Can you work these out from the model? Positions are in its coordinate system, mm. A direction names the side the tool comes from. Coordinates: 2 decimals unless noted, no trailing zeros. Loops run counter-clockwise (first coordinate to the right, second up) from the corner with the lowest first, then second, coordinate; pieces in that order, holes last.
Autodesk Fusion 360 part; units mm, degrees
sketch "草图1" plane through (0, 0, 0) normal (0, 1, 0) x (1, 0, 0)
  line L0 (-100, 0) -> (100, 0) construction
  line L1 (-50, 0) -> (-50, -14)
  line L2 (-50, -14) -> (-26.533, -14)
  arc A0 (-26.533, -14) -> (26.533, -14) centre (0, 0) ccw
  line L3 (26.533, -14) -> (50, -14)
  line L4 (50, -14) -> (50, 0)
  line L5 (18, 0) -> (50, 0)
  line L6 (-50, 0) -> (-18, 0)
  line L7 (0, -85) -> (0, 30) construction
  arc A1 (-18, 0) -> (18, 0) centre (0, 0) ccw
  circle A2 centre (0, -60) radius 16
  circle A3 centre (0, -60) radius 9
  line L8 (-26.533, -14) -> (-15.6243, -63.4469)
  line L9 (26.533, -14) -> (15.6243, -63.4469)
  line L10 (-21.2383, -38) -> (21.2383, -38)
  dimension "d1" = 14
  dimension "d2" = 14
  dimension "d3" = 100
  dimension "d5" = 30
  dimension "d6" = 18
  dimension "d7" = 32
  dimension "d8" = 18
  dimension "d9" = 60
  dimension "d10" = 38
extrude "拉伸1" add sketch "草图1" against normal blind 50 contours L1 L2 A0 L3 L4 L5 L6 A1 makes body 1
extrude "拉伸2" add sketch "草图1" against normal blind 45 contours A0 L8 L9 L10 bodies 1
extrude "拉伸3" add sketch "草图1" against normal blind 15 contours A2 L8 L9 L10 bodies 1
extrude "拉伸4" add sketch "草图1" against normal blind 17 contours A2 bodies 1
sketch "草图2" plane through (0, 0, 0) normal (1, 0, 0) x (0, 1, 0)
  line L0 (-15, 63.4469) -> (-15, 41)
  line L1 (-18, 38) -> (-45, 38)
  arc A0 (-18, 38) -> (-15, 41) centre (-18, 41) ccw
  line L2 (-15, 63.4469) -> (-15, 38)
  line L3 (-15, 38) -> (-45, 38)
  point P0 (-15, 63.4469)
  point P1 (-45, 38)
  point P2 (-15, 38)
  dimension "d19" = 3
extrude "拉伸5" add sketch "草图2" along normal mid plane 54 separate body makes body 2
extrude "拉伸6" cut sketch "草图1" against normal blind 75 contours A2 L8 L9 L10 keep common part bodies 2
combine "合并1" operation add target body 1 tool bodies 2
sketch "草图3" plane through (0, 0, 0) normal (0, 0, 1) x (1, 0, 0)
  line L0 (-50, -17) -> (-50, -33)
  line L1 (-50, -33) -> (-36, -33)
  arc A0 (-36, -33) -> (-36, -17) centre (-36, -25) ccw
  line L2 (-36, -17) -> (-50, -17)
  line L3 (0, 15) -> (0, -36) construction
  line L4 (36, -17) -> (50, -17)
  line L5 (50, -17) -> (50, -33)
  line L6 (50, -33) -> (36, -33)
  arc A1 (36, -17) -> (36, -33) centre (36, -25) ccw
  dimension "d24" = 50
  dimension "d25" = 36
  dimension "d26" = 16
  dimension "d27" = 25
extrude "拉伸7" cut sketch "草图3" along normal blind 14 bodies 1
sketch "草图4" plane through (0, 0, 38) normal (0, 0, 1) x (-1, 0, 0)
  line L0 (-21.2383, 18) -> (21.2383, 18)
  line L1 (21.2383, 18) -> (21.2383, 45)
  line L2 (21.2383, 45) -> (-21.2383, 45)
  line L3 (-21.2383, 45) -> (-21.2383, 18)
  circle A0 centre (0, 30) radius 5
  line L4 (0, 45) -> (0, 18) construction
  dimension "d30" = 15
  dimension "d31" = 10
extrude "拉伸8" cut sketch "草图4" against normal blind 57 contours A0 bodies 1
equation "d10 = 60 mm - 22 mm"
(1) I want a section at A-A on x = -40. Write out the boundary of the cut face in (y, z).
Check values:
outline: (-50, 0) - (-33, 0) - (-33, 14) - (-50, 14) - close; (-17, 0) - (0, 0) - (0, 14) - (-17, 14) - close
(2) I want a section at C-C on z = 60. Write out the boundary of the cut face in (x, y), then the cut area to 3 significant figures.
Check values:
outline: (-16.38, -15) - (-16, -15) - (-16, -17) - (-9, -17) - (-9, 0) - (-16.38, 0) - close; (9, -17) - (16, -17) - (16, -15) - (16.38, -15) - (16.38, 0) - (9, 0) - close
area: 250 mm2
(3) I want a section at D-D on y = -30. Write out the boundary of the cut face in (x, z) (3 decimals).
Check values:
outline: (-29.755, 0) - (-18, 0) arc R18 cw to (-5, 17.292) - (-5, 38) - (-21.238, 38) - (-26.533, 14) - (-29.755, 14) - close; (5, 17.292) arc R18 cw to (18, 0) - (29.755, 0) - (29.755, 14) - (26.533, 14) - (21.238, 38) - (5, 38) - close
(4) I'm going to push flat-ended pins straight in: pin 1 (23.5 mm diameter, centred on x = 0, z = 60, fed in from -Y); pin 2 (7 mm diameter, centred on x = 37, y = -18, fed in from +Z); pin 3 (2 mm diameter, centred on y = -15.5, z = 65, fed in from -X); pin 4 (1 mm diameter, centred on x = 16, z = 66, fed in from +Y). Where does each tip first touch, or does it pass through?
Check values:
pin 1: stops at y = -17
pin 2: stops at z = 14
pin 3: stops at x = -15.49
pin 4: passes through
(5) Which directions (+Z, -Z, +X, -X, +Y, -Y) give clear straight access to the entire face, cutting with the end or side of a thin tool? Please do faces 1 (the flat face through (30, -19, 14)), 2 (the flat face through (-38, -14, 14)), 3 (the cylindrical face through (-3.47, -8.38, 75.62)), 4 (the flat face through (-5, -31.3, 38)).
Check values:
face 1: +Z, +X, +Y, -Y
face 2: +Z, -X, +Y, -Y
face 3: -Y
face 4: +Z, +X, -X, -Y
(6) I want a section at B-B on x = 0. Write out the boundary of the cut face in (y, z).
Check values:
outline: (-50, 18) - (-35, 18) - (-35, 38) - (-45, 38) - (-45, 30) - (-50, 30) - close; (-25, 18) - (0, 18) - (0, 51) - (-17, 51) - (-17, 44) - (-15, 44) - (-15, 41) arc R3 cw to (-18, 38) - (-25, 38) - close; (-17, 69) - (0, 69) - (0, 76) - (-17, 76) - close
(7) If we mould it in two halves opening along Y, with no side actions, what happens to faces 5 (the cylindrical face through (28, -25, 7)), 6 (the flat face through (0, -45, 31)), 7 (the flat face through (50, -8, 7))? For each: released by +Y, released by -Y, zero draft, split by the parting line, or undercut.
Check values:
face 5: undercut
face 6: released by -Y
face 7: zero draft
(8) If I drill on probe 1 along Y at (x, z) = (38, 12); probe 2 along Z at (x, y) = (0, -11.25); probe 3 along X at (y, z) = (-9, 9), over which ranges is the centre line in solid material (lowest first)?
Check values:
probe 1: y = -50 to -33, -17 to 0
probe 2: z = 18 to 51, 69 to 76
probe 3: x = -50 to -15.59, 15.59 to 50
